```python
from build123d import *

# Parameters (mm, degrees)
SKETCH1_R           = 12.7
BOSS_EXTRUDE1_DEPTH = 8.89
SKETCH2_R           = 2.54
CUT_EXTRUDE1_DEPTH  = 6.35
FILLET1_R           = 2.54


with BuildPart() as part:
    # Sketch1 → Boss-Extrude1 (new body)
    with BuildSketch(Plane.XY):
        Circle(SKETCH1_R)
    extrude(amount=BOSS_EXTRUDE1_DEPTH)

    # Sketch2 → Cut-Extrude1 (cut)
    with BuildSketch(Plane(origin=(0, 0, 0), x_dir=(-1, 0, 0), z_dir=(0, 0, -1))):
        Circle(SKETCH2_R)
    extrude(amount=-CUT_EXTRUDE1_DEPTH, mode=Mode.SUBTRACT)

    # Fillet1
    fillet1_edges = [part.edges().sort_by_distance(p)[0] for p in [
        (-12.7, 0, 0),
        (-12.7, 0, 8.89),
    ]]
    fillet(fillet1_edges, radius=FILLET1_R)


solid = part.part
```
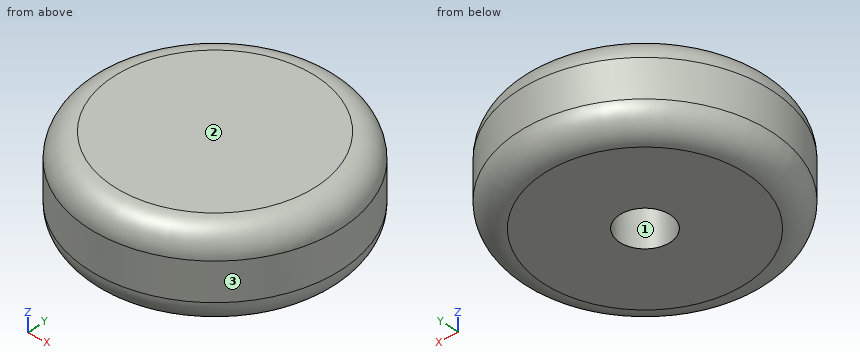
Build history of the part. All positions in model axes, mm. Face numbers are marked on the shaded views. Coordinates: 2 decimals unless noted, no trailing zeros. Order: outer loops, then holes, each group sorted by start corner. A loop starts at its lowest first (then second) coordinate and runs counter-clockwise, first axis right, second up.
Item 1: Drop flat-ended pins along their axis: pin 1 Ø4 at (x, z) = (4, 2) entering from -Y; pin 2 Ø1.5 at (x, z) = (5, 2.5) entering from -Y; pin 3 Ø5 at (x, z) = (3, 7.5) entering from +Y. Give the stop position or say it passes through.
Filled in:
pin 1: stops at y = -12.53
pin 2: stops at y = -11.97
pin 3: stops at y = 12.68
Item 2: Saw through at C-C on z = 5. List the corners of the cut face in (x, y).
Filled in:
outline: circle Ø25.4 at (0, 0); hole circle Ø5.08 at (0, 0)
Item 3: Saw through at D-D on z = 2. List the corners of the cut face in (x, y), then the cut area to 3 significant figures.
Filled in:
outline: circle Ø25.28 at (0, 0); hole circle Ø5.08 at (0, 0)
area: 482 mm2
Item 4: Saw through at A-A on y = 0. List the corners of the cut face in (x, z), then the cut area to 3 significant figures.
Filled in:
outline: (-12.7, 2.54) arc R2.54 ccw to (-10.16, 0) - (-2.54, 0) - (-2.54, 6.35) - (2.54, 6.35) - (2.54, 0) - (10.16, 0) arc R2.54 ccw to (12.7, 2.54) - (12.7, 6.35) arc R2.54 ccw to (10.16, 8.89) - (-10.16, 8.89) arc R2.54 ccw to (-12.7, 6.35) - close
area: 188 mm2
Item 5: Mould opens along Y. For the marked faces 1, 2 and 3 say: released by +Y, released by -Y, zero draft, split by the parting line, or undercut.
Filled in:
face 1: undercut
face 2: zero draft
face 3: split by the parting line
Item 6: Drill centre lines: L1, parallel to Y at x = 0, z = 2.5; L2, parallel to Y at x = 0, z = 2; L3, parallel to X at y = -0.5, z = 4.5. Where is each one in solid material? Low to high.
Filled in:
L1: y = -12.7 to -2.54, 2.54 to 12.7
L2: y = -12.64 to -2.54, 2.54 to 12.64
L3: x = -12.69 to -2.49, 2.49 to 12.69
